```python
from build123d import *

# Parameters (mm, degrees)
F0_R     = 4.7625
F0_R_2   = 2.3749
F1_DEPTH = 9.525
F2_R     = 0.254
F3_R     = 0.254


with BuildPart() as f1:
    # F0 (on Front) → F1 (new body)
    with BuildSketch(Plane.XZ):
        Circle(F0_R)
        Circle(F0_R_2, mode=Mode.SUBTRACT)
    extrude(amount=F1_DEPTH)

    # F2
    f2_edges = [f1.edges().sort_by_distance(p)[0] for p in [
        (-4.7625, -9.525, 0),
        (-4.7625, 0, 0),
    ]]
    fillet(f2_edges, radius=F2_R)

    # F3
    f3_edges = [f1.edges().sort_by_distance(p)[0] for p in [
        (-2.3749, -9.525, 0),
        (-2.3749, 0, 0),
    ]]
    fillet(f3_edges, radius=F3_R)


solid = f1.part
```
Can you work these out from the model? Positions are in its coordinate system, mm. Coordinates: 2 decimals unless noted, no trailing zeros. Loops run counter-clockwise (first coordinate to the right, second up) from the corner with the lowest first, then second, coordinate; pieces in that order, holes last. Notation, with made-up numbers: M 35.5,64.25 L 75.5,64.25 A9 ccw 75.5,70.25 Z; hole C 88,67 d11. An arc over 180 degrees is marked long. Put each result on its own line as item: value. Start each with the question number.
(1) I need wall thicknesses on probe 1 along Z at (x, y) = (0, -7.75); probe 2 along Z at (x, y) = (-0.5, -4); probe 3 along X at (y, z) = (-4.5, 1.25). Which ranges of each line are inside material? Lowest first, please.
(2) We'd pull the mould along X, two halves only. Please class faces 1 (the face through (-1.75, -4.699, 1.605)), 2 (the face through (2, 0, -2)), 3 (the face through (-3.78, -4.7, -2.9)): +X half, -X half, draft (parallel to the pull), parting line (faces both ways), or undercut.
(3) Will these pins go through, and if not, where does the flat tip stop? pin 1 Ø1.5 at (x, y) = (-1, -1.5) entering from +Z; pin 2 Ø3 at (y, z) = (-6.5, 2) entering from +X; pin 3 Ø1 at (x, y) = (-2, -3) entering from +Z.
(4) Imagine slicing it at C-C on y = -7. List the corners of the cut face in (x, z) for me (1 decimal).
Worked answers:
1. probe 1: z = -4.76 to -2.37, 2.37 to 4.76
1. probe 2: z = -4.74 to -2.32, 2.32 to 4.74
1. probe 3: x = -4.6 to -2.02, 2.02 to 4.6
2. face 1: undercut
2. face 2: draft
2. face 3: parting line
3. pin 1: stops at z = 4.76
3. pin 2: stops at x = 4.74
3. pin 3: stops at z = 4.52
4. outline: C 0,0 d9.5; hole C 0,0 d4.7
